Check sheet for the modelled part. Datum: model origin and axes. Units: mm. Face numbers are marked on the shaded views. Round coordinates to 2 decimals unless told otherwise and drop trailing zeros. Order: outer loops, then holes, each group sorted by start corner. A loop starts at its lowest first (then second) coordinate and runs counter-clockwise, first axis right, second up. Notation, with made-up numbers: (47.25, 52) -> (106.25, 52) arc R15 ccw to (106.25, 59) -> close; hole circle Ø10 at (44.25, 62.25). An arc over 180 degrees is marked (long way). Answer in a Markdown table with one row per item.
from build123d import *

# Parameters (mm, degrees)
SKETCH1_R           = 1.5
BOSS_EXTRUDE1_DEPTH = 8


with BuildPart() as part:
    # Sketch1 → Boss-Extrude1 (new body)
    with BuildSketch(Plane(origin=(0, 0, 0), x_dir=(1, 0, 0), z_dir=(0, 1, 0))):
        Polygon((0, 2), (0.487725805, 2.451963201), (0.765366865, 1.847759065), (1.388925583, 2.078674031), (1.414213562, 1.414213562), (2.078674031, 1.388925583), (1.847759065, 0.765366865), (2.451963201, 0.487725805), (2, 0), (2.451963201, -0.487725805), (1.847759065, -0.765366865), (2.078674031, -1.388925583), (1.414213562, -1.414213562), (1.388925583, -2.078674031), (0.765366865, -1.847759065), (0.487725805, -2.451963201), (0, -2), (-0.487725805, -2.451963201), (-0.765366865, -1.847759065), (-1.388925583, -2.078674031), (-1.414213562, -1.414213562), (-2.078674031, -1.388925583), (-1.847759065, -0.765366865), (-2.451963201, -0.487725805), (-2, 0), (-2.451963201, 0.487725805), (-1.847759065, 0.765366865), (-2.078674031, 1.388925583), (-1.414213562, 1.414213562), (-1.388925583, 2.078674031), (-0.765366865, 1.847759065), (-0.487725805, 2.451963201), align=None)
        Circle(SKETCH1_R, mode=Mode.SUBTRACT)
    extrude(amount=BOSS_EXTRUDE1_DEPTH)


solid = part.part
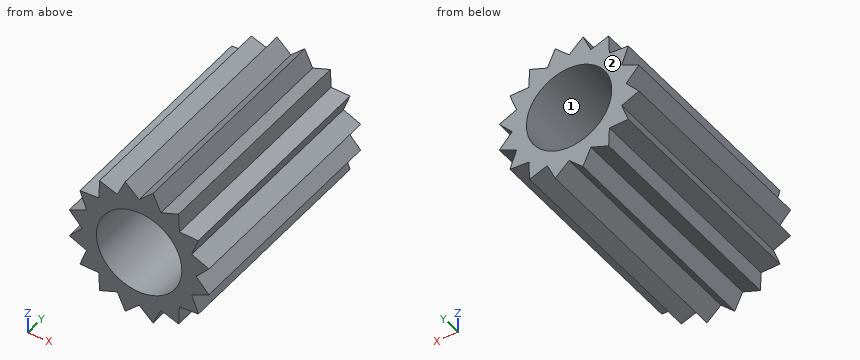
Item 1: Scan lines: line 1 (X direction, y = 4.5, z = 0.1); line 2 (X direction, y = 2.5, z = 1.15); line 3 (Z direction, x = -1.05, y = 0.75). Record each from-to range of solid material in increasing order. Write a range as [from, to].
Result sheet:
| item | result |
|---|---|
| line 1 | x = [-2.09, -1.5], [1.5, 2.09] |
| line 2 | x = [-1.99, -0.96], [0.96, 1.99] |
| line 3 | z = [-1.95, -1.07], [1.07, 1.95] |
Item 2: Cross-section at C-C (z = -1.1). Record the boundary of the cut face in (x, y).
Result sheet:
| item | result |
|---|---|
| outline | (-1.97, 0) -> (-1.02, 0) -> (-1.02, 8) -> (-1.97, 8) -> close; (1.02, 0) -> (1.97, 0) -> (1.97, 8) -> (1.02, 8) -> close |
Item 3: Mould release check, pull along X, two halves, no side actions. Record for the marked faces 1 and 2: pulls with the +X half, pulls with the -X half, needs draft (parallel to the pull), parting line crosses it, or undercut.
Result sheet:
| item | result |
|---|---|
| face 1 | undercut |
| face 2 | needs draft |
Item 4: Depth check by flat-ended pin: P1, Ø1.5, axis at y = 1, z = 1.5, coming from the +X side. Enter the tip coordinate at first touch or a pass-through.
Result sheet:
| item | result |
|---|---|
| P1 | stops at x = 2.08 |
Item 5: Cross-section at B-B (x = -1.2). Record the boundary of the cut face in (y, z).
Result sheet:
| item | result |
|---|---|
| outline | (0, -2.01) -> (8, -2.01) -> (8, -0.9) -> (0, -0.9) -> close; (0, 0.9) -> (8, 0.9) -> (8, 2.01) -> (0, 2.01) -> close |
